Geometry check sheet. Reference: the model listing, model coordinates, mm. A direction names the side the tool comes from. Coordinates: 2 decimals unless noted, no trailing zeros. Write each loop counter-clockwise with the first axis right and the second up, starting at its lowest first coordinate (ties: lowest second). Pieces come first, ordered by that corner, then holes. Notation, with made-up numbers: (10.25, -7.75) -> (31.25, -7.75) arc R15 cw to (31.25, 13.25) -> close; hole circle Ø3 at (68.25, 77). An arc over 180 degrees is marked (long way). Answer in a Markdown table with one row per item. Add a question column.
Q1. Gauge pin test, flat ends, axial feed: P1, Ø18, axis at y = 9, z = 0, coming from the -X side; P2, Ø10, axis at x = -2.5, y = -7, coming from the -Z side; P3, Ø10, axis at x = 2.5, z = -10.5, coming from the -Y side. Record the tip position at first contact, or that the pin passes through.
Q2. Release check for a two-part mould opening along X. For faces 1 (the face through (0.2, 16.4, -19.1)), 2 (the face through (-10.1, -15, 0)), 3 (the face through (13, -6, 0)) record: pulls with the +X half, pulls with the -X half, needs draft (parallel to the pull), parting line crosses it, or undercut.
Q3. Section check D-D, the plane z = -16.5. Record the boundary of the cut face in (x, y), and give its area (3 significant figures).
Q4. Thickness scan on line 1 (Y direction, x = 0.5, z = 0); line 2 (Z direction, x = 8.75, y = 9.5); line 3 (X direction, y = -14, z = -14). Record the ranges inside material, lowest first.
Q5. Section check B-B, the plane x = -5.5. Record the boundary of the cut face in (y, z), and give its area (3 significant figures).
Q6. Section check A-A, the plane y = -18.5. Record the boundary of the cut face in (x, z), and give its area (3 significant figures).
Q7. Tool access check on faces 4 (the face through (0, -4.8, 0)), 5 (the face through (0, 1, 25)). Record the directions out of +Z, -Z, +X, -X, +Y, -Y that give a thin tool (end or side, any length) a straight path to the whole face; none if there is none.
Q8. Section check C-C, the plane z = 0. Record the boundary of the cut face in (x, y).
```python
from build123d import *

# Parameters (mm, degrees)
SKETCH_1_R          = 11.25
EXTRUDE_1_DEPTH     = 13
SKETCH_2_W          = 20.2
SKETCH_2_H          = 20.2
CUT_EXTRUDE_1_DEPTH = 58.393379409


with BuildPart() as part:
    # Эскиз1 → Бобышка-Вытянуть1 (new, symmetric)
    with BuildSketch(Plane(origin=(0, 0, 0), x_dir=(0, 0, -1), z_dir=(1, 0, 0))):
        Polygon((-25, -25), (25, -25), (25, 10.5), (13, 22.5), (-13, 22.5), (-25, 10.5), align=None)
        with Locations(Location((0, 9, 0), (0, 0, 180))):
            Circle(SKETCH_1_R, mode=Mode.SUBTRACT)
    extrude(amount=EXTRUDE_1_DEPTH, both=True)

    # Эскиз2 → Вырез-Вытянуть1 (cut, through all)
    with BuildSketch(Plane(origin=(0, 0, -25), x_dir=(-1, 0, 0), z_dir=(0, 0, -1))):
        with Locations((0, -14.9)):
            Rectangle(SKETCH_2_W, SKETCH_2_H)
    extrude(amount=-CUT_EXTRUDE_1_DEPTH, mode=Mode.SUBTRACT)


solid = part.part
```
Calculated:
| question | item | result |
|---|---|---|
| 1 | P1 | passes through |
| 1 | P2 | stops at z = -25 |
| 1 | P3 | stops at y = -4.8 |
| 2 | face 1 | needs draft |
| 2 | face 2 | undercut |
| 2 | face 3 | pulls with the +X half |
| 3 | outline | (-13, -25) -> (-10.1, -25) -> (-10.1, -4.8) -> (10.1, -4.8) -> (10.1, -25) -> (13, -25) -> (13, 19) -> (-13, 19) -> close |
| 3 | area | 736 mm² |
| 4 | line 1 | y = -4.8 to -2.25, 20.25 to 22.5 |
| 4 | line 2 | z = -25 to -11.24, 11.24 to 25 |
| 4 | line 3 | x = -13 to -10.1, 10.1 to 13 |
| 5 | outline | (-4.8, -25) -> (10.5, -25) -> (22.5, -13) -> (22.5, 13) -> (10.5, 25) -> (-4.8, 25) -> close; hole circle Ø22.5 at (9, 0) |
| 5 | area | 823 mm² |
| 6 | outline | (-13, -25) -> (-10.1, -25) -> (-10.1, 25) -> (-13, 25) -> close; (10.1, -25) -> (13, -25) -> (13, 25) -> (10.1, 25) -> close |
| 6 | area | 290 mm² |
| 7 | face 4 | +Z, -Z, -Y |
| 7 | face 5 | +Z, +X, -X, +Y, -Y |
| 8 | outline | (-13, -25) -> (-10.1, -25) -> (-10.1, -4.8) -> (10.1, -4.8) -> (10.1, -25) -> (13, -25) -> (13, -2.25) -> (-13, -2.25) -> close; (-13, 20.25) -> (13, 20.25) -> (13, 22.5) -> (-13, 22.5) -> close |
